Input: part model. Units: mm. Frame: model coordinates. A direction names the side the tool comes from. Round coordinates to 2 decimals unless told otherwise and drop trailing zeros. Write each loop counter-clockwise with the first axis right and the second up, starting at its lowest first coordinate (ties: lowest second). Pieces come first, ordered by that corner, then holes. Notation, with made-up numbers: (-4, 79.5) - (11, 79.5) arc R20 ccw to (11, 105.5) - close; hole circle Ø9 at (-1.75, 56). An arc over 180 degrees is marked (long way). One line per item, written item: value. Start each with the question number.
```python
from build123d import *

# Parameters (mm, degrees)
BOSS_EXTRUDE1_DEPTH     = 25.6
SKETCH2_W               = 4.3
SKETCH2_H               = 15.7
CUT_EXTRUDE1_DEPTH      = 3
CUT_EXTRUDE2_REACH      = 52.281
SKETCH3_R               = 1.3
BOSS_EXTRUDE2_START     = -1.6
BOSS_EXTRUDE2_DEPTH     = 1.6
SKETCH6_W               = 20
SKETCH6_H               = 1.7
BOSS_EXTRUDE3_DEPTH     = 3
CHAMFER2_SIZE           = 3
BOSS_EXTRUDE5_DEPTH     = 17
CHAMFER3_SIZE           = 1.6
CUT_EXTRUDE3_REACH      = 52.926
SKETCH9_W               = 18.51367302
SKETCH9_H               = 5.5
LPATTERN1_COUNT         = 4
LPATTERN1_PITCH         = 7
CUT_EXTRUDE4_REACH      = 53.699
SKETCH10_W              = 21
SKETCH10_H              = 4
LPATTERN2_COUNT         = 4
LPATTERN2_PITCH         = 6
SKETCH11_W              = 4.3
SKETCH11_H              = 15.7
CUT_EXTRUDE5_DEPTH      = 20
CHAMFER4_SIZE           = 4.2
CUT_EXTRUDE6_REACH      = 54.653
SKETCH12_W              = 15.8
SKETCH12_H              = 4
LPATTERN3_COUNT         = 3
LPATTERN3_PITCH         = 6
CUT_EXTRUDE7_REACH      = 55.459
CUT_EXTRUDE7_END_RADIUS = 10.65
SKETCH13_W              = 21
SKETCH13_H              = 3.317301245


# Some blends are built 0.0001 mm under size
with BuildPart() as part:
    # Sketch1 → Boss-Extrude1 (new body)
    with BuildSketch(Plane(origin=(0, 0, 0), x_dir=(0, 0, -1), z_dir=(1, 0, 0))):
        with BuildLine():
            Line((-2, 32), (-2, 30))
            Line((-2, 30), (0, 30))
            Line((0, 30), (0, 34))
            Line((0, 34), (-17.35, 34))
            ThreePointArc((-17.35, 34), (-25.835281374, 30.485281374), (-29.35, 22))
            Line((-29.35, 22), (-29.35, 0))
            Line((-29.35, 0), (-23.7, 0))
            Line((-23.7, 0), (-23.7, 15.7))
            Line((-23.7, 15.7), (-28, 15.7))
            Line((-28, 15.7), (-28, 22))
            ThreePointArc((-28, 22), (-26.080424321, 28.099359898), (-21.01367302, 32))
            Line((-21.01367302, 32), (-2, 32))
        make_face()
    extrude(amount=-BOSS_EXTRUDE1_DEPTH)

    # Sketch2 → Cut-Extrude1 (cut)
    with BuildSketch(Plane(origin=(0, 0, 0), x_dir=(0, 0, -1), z_dir=(1, 0, 0))):
        with Locations((-25.85, 7.85)):
            Rectangle(SKETCH2_W, SKETCH2_H)
    extrude(amount=-CUT_EXTRUDE1_DEPTH, mode=Mode.SUBTRACT)

    # Sketch3 → Cut-Extrude2 (cut, up to next)
    with BuildSketch(Plane(origin=(-3, 0, 0), x_dir=(0, 0, -1), z_dir=(1, 0, 0)), mode=Mode.PRIVATE) as cut_extrude2_sk1:
        with Locations((-25.65, 9.5)):
            Circle(SKETCH3_R)
    cut_extrude2_tool1 = extrude(cut_extrude2_sk1.sketch, amount=-CUT_EXTRUDE2_REACH, mode=Mode.PRIVATE) & part.part
    add(cut_extrude2_tool1.solids().sort_by_distance((-3, 9.5, 25.65))[0], mode=Mode.SUBTRACT)

    # Sketch4 → Boss-Extrude2 (add)
    with BuildSketch(Plane.ZY.offset(25.6).offset(BOSS_EXTRUDE2_START)):
        with BuildLine():
            Line((0, 34), (0, 0))
            Line((0, 0), (29.35, 0))
            Line((29.35, 0), (29.35, 22))
            ThreePointArc((29.35, 22), (25.835281374, 30.485281374), (17.35, 34))
            Line((17.35, 34), (0, 34))
        make_face()
    extrude(amount=BOSS_EXTRUDE2_DEPTH)

    # Sketch6 → Boss-Extrude3 (add)
    with BuildSketch(Plane(origin=(0, 0, 0), x_dir=(-1, 0, 0), z_dir=(0, 0, -1))):
        with Locations((10, 30.85)):
            Rectangle(SKETCH6_W, SKETCH6_H)
    extrude(amount=BOSS_EXTRUDE3_DEPTH)

    # Chamfer2
    chamfer2_edges = [part.edges().sort_by_distance(p)[0] for p in [
        (-20, 30.85, -3),
    ]]
    chamfer(chamfer2_edges, length=CHAMFER2_SIZE - 0.0001)  # a hair under: the kernel refuses the full size

    # Sketch8 → Boss-Extrude5 (add)
    with BuildSketch(Plane.ZY):
        Polygon((-1.408034607, 31.7), (-1.808034607, 33.3), (-3, 33.3), (-3, 31.7), align=None)
    extrude(amount=BOSS_EXTRUDE5_DEPTH)

    # Chamfer3
    chamfer3_edges = [part.edges().sort_by_distance(p)[0] for p in [
        (-17, 33.3, -2.404017304),
    ]]
    chamfer(chamfer3_edges, length=CHAMFER3_SIZE - 0.0001)  # a hair under: the kernel refuses the full size

    # Sketch9 → Cut-Extrude3 (cut, up to next)
    with BuildSketch(Plane(origin=(-24, 0, 0), x_dir=(0, 0, -1), z_dir=(1, 0, 0)), mode=Mode.PRIVATE) as cut_extrude3_sk1:
        with Locations((-13.25683651, 27.25)):
            Rectangle(SKETCH9_W, SKETCH9_H)
    cut_extrude3_tool1 = extrude(cut_extrude3_sk1.sketch, amount=-CUT_EXTRUDE3_REACH, mode=Mode.PRIVATE) & part.part
    cut_extrude3 = cut_extrude3_tool1.solids().sort_by_distance((-24, 27.25, 13.256837))[0]
    add(cut_extrude3, mode=Mode.SUBTRACT)

    # LPattern1: Cut-Extrude3 ×4
    with Locations(*[(0, -i * LPATTERN1_PITCH, 0) for i in range(1, LPATTERN1_COUNT)]):
        add(cut_extrude3, mode=Mode.SUBTRACT)

    # Sketch10 → Cut-Extrude4 (cut, up to next)
    with BuildSketch(Plane(origin=(0, 34, 0), x_dir=(1, 0, 0), z_dir=(0, 1, 0)), mode=Mode.PRIVATE) as cut_extrude4_sk1:
        with Locations((-13.5, -6)):
            Rectangle(SKETCH10_W, SKETCH10_H)
    cut_extrude4_tool1 = extrude(cut_extrude4_sk1.sketch, amount=-CUT_EXTRUDE4_REACH, mode=Mode.PRIVATE) & part.part
    cut_extrude4 = cut_extrude4_tool1.solids().sort_by_distance((-13.5, 34, 6))[0]
    add(cut_extrude4, mode=Mode.SUBTRACT)

    # LPattern2: Cut-Extrude4; each copy of Cut-Extrude4 runs up to whatever stops it at its own place
    lpattern2_before = part.part  # the part as the pattern finds it: every copy runs up to it
    lpattern2_cut_extrude4_long = extrude(cut_extrude4_sk1.sketch, amount=-CUT_EXTRUDE4_REACH, mode=Mode.PRIVATE)
    lpattern2_cut_extrude4_tool1 = lpattern2_cut_extrude4_long.moved(Location(Vector(0, 0, 1) * (1 * LPATTERN2_PITCH))) & lpattern2_before
    add(lpattern2_cut_extrude4_tool1.solids().sort_by_distance((-13.5, 34, 12))[0], mode=Mode.SUBTRACT)
    lpattern2_cut_extrude4_tool2 = lpattern2_cut_extrude4_long.moved(Location(Vector(0, 0, 1) * (2 * LPATTERN2_PITCH))) & lpattern2_before
    add(lpattern2_cut_extrude4_tool2.solids().sort_by_distance((-13.5, 34, 18))[0], mode=Mode.SUBTRACT)
    lpattern2_cut_extrude4_tool3 = lpattern2_cut_extrude4_long.moved(Location(Vector(0, 0, 1) * (3 * LPATTERN2_PITCH))) & lpattern2_before
    add(lpattern2_cut_extrude4_tool3.solids().sort_by_distance((-13.5, 34, 24))[0], mode=Mode.SUBTRACT)

    # Sketch11 → Cut-Extrude5 (cut)
    with BuildSketch(Plane(origin=(-24, 0, 0), x_dir=(0, 0, -1), z_dir=(1, 0, 0))):
        with Locations((-25.85, 7.85)):
            Rectangle(SKETCH11_W, SKETCH11_H)
    extrude(amount=CUT_EXTRUDE5_DEPTH, mode=Mode.SUBTRACT)

    # Chamfer4
    # the kernel refuses this chamfer: 4.2 mm, written as the material it adds along each edge
    with BuildSketch(Plane(origin=(-4, 15.7, 28), x_dir=(-0.9996219169112966, 0, 0.02749587661058612), z_dir=(0, -1, 0))) as chamfer4_piece_1_section:
        Polygon((CHAMFER4_SIZE * 0.999621916911, CHAMFER4_SIZE * 0.0274958766106), (-CHAMFER4_SIZE * 0.0274958766106, CHAMFER4_SIZE * 0.999621916911), (0, 0), align=None)
    chamfer4_piece_1 = extrude(amount=15.7, mode=Mode.PRIVATE)
    chamfer4_piece_1 = chamfer4_piece_1 - Plane(origin=(-5.414149403, 9.5, 25.65), x_dir=(0, 0, -1), z_dir=(1, 0, 0)) * Cylinder(1.3, 49, mode=Mode.PRIVATE)
    add(chamfer4_piece_1)

    # Sketch12 → Cut-Extrude6 (cut, up to next)
    with BuildSketch(Plane(origin=(0, 0, 28), x_dir=(-1, 0, 0), z_dir=(0, 0, -1)), mode=Mode.PRIVATE) as cut_extrude6_sk1:
        with Locations((16.1, 5.5)):
            Rectangle(SKETCH12_W, SKETCH12_H)
    cut_extrude6_tool1 = extrude(cut_extrude6_sk1.sketch, amount=-CUT_EXTRUDE6_REACH, mode=Mode.PRIVATE) & part.part
    cut_extrude6 = cut_extrude6_tool1.solids().sort_by_distance((-16.1, 5.5, 28))[0]
    add(cut_extrude6, mode=Mode.SUBTRACT)

    # LPattern3: Cut-Extrude6 ×3
    with Locations(*[(0, i * LPATTERN3_PITCH, 0) for i in range(1, LPATTERN3_COUNT)]):
        add(cut_extrude6, mode=Mode.SUBTRACT)

    # Cut-Extrude7: up to this cylinder (the profile starts outside it)
    cut_extrude7_end = Plane(origin=(-13.5, 22, 17.35), z_dir=(1, 0, 0)) * Cylinder(CUT_EXTRUDE7_END_RADIUS, 133.218, mode=Mode.PRIVATE)
    # Sketch13 → Cut-Extrude7 (cut, up to the surface)
    with BuildSketch(Plane.XY.offset(29.35), mode=Mode.PRIVATE) as cut_extrude7_sk1:
        with Locations((-13.5, 26.158650623)):
            Rectangle(SKETCH13_W, SKETCH13_H)
    cut_extrude7_tool1 = extrude(cut_extrude7_sk1.sketch, amount=-CUT_EXTRUDE7_REACH, mode=Mode.PRIVATE) - cut_extrude7_end
    add(cut_extrude7_tool1.solids().sort_by_distance((-13.5, 26.158651, 29.35))[0], mode=Mode.SUBTRACT)


solid = part.part
```
Q1. Contact query for flat-ended pins moving along their axis: pin 1 Ø8 at (y, z) = (7, 19) entering from +X; pin 2 Ø1.2 at (x, y) = (-12.5, 32.5) entering from +Z; pin 3 Ø15 at (x, z) = (-10, 12) entering from -Y; pin 4 Ø1 at (y, z) = (12.5, 13.5) entering from +X. Output: stop coordinate, or through.
Q2. Access query for faces 1 (the flat face through (-14, 33, 20)), 2 (the flat face through (-25, 24.5, 13)), 3 (the flat face through (-11.8, 32, 9.5)). Directions: +Z, -Z, +X, -X, +Y, -Y. A direction counts if a zero-diameter tool reaches every point of the face in a straight line with its end or side. Return the directions, or none.
Q3. Cut plane D-D, the plane x = -3.5. Count the separate pieces of the cut face and the enclosed holes in it, and give its area (3 significant figures).
Q4. Cut plane A-A, the plane z = 14.5. Output: boundary loops of the cut face in (x, y).
Q5. Cut plane B-B, the plane y = 7. Output: boundary loops of the cut face in (x, z).
Q6. Material intervals for probe 1 along Y at (x, z) = (-5.75, 25.65); probe 2 along Z at (x, y) = (-4.4, 9.5); probe 3 along X at (y, z) = (1, 25), sorted ascending. Write a range as from..to.
Q7. Pull-direction query (Y, two-part tool) for faces 4 (the flat face through (-3, 33, 18)), 5 (the flat face through (-8.381, 32.489, -1.605)), 6 (the flat face through (-25, 10.5, 13)); classes: pulls with the +Y half, pulls with the -Y half, needs draft (parallel to the pull), parting line crosses it, or undercut.
Q8. Cut plane C-C, the plane y = 21. Output: boundary loops of the cut face in (x, z), and give its area (3 significant figures).
A:
1. pin 1: stops at x = -24
1. pin 2: stops at z = 22
1. pin 3: stops at y = 32
1. pin 4: passes through
2. face 1: +Y, -Y
2. face 2: +X, -X
2. face 3: +X, -Y
3. separate pieces: 6
3. enclosed holes: 1
3. area: 128 mm²
4. outline: (-25.6, 0) - (-24, 0) - (-24, 3.5) - (-25.6, 3.5) - close; (-25.6, 9) - (-24, 9) - (-24, 10.5) - (-25.6, 10.5) - close; (-25.6, 16) - (-24, 16) - (-24, 17.5) - (-25.6, 17.5) - close; (-25.6, 23) - (-24, 23) - (-24, 24.5) - (-25.6, 24.5) - close; (-25.6, 30) - (-24, 30) - (-24, 32) - (0, 32) - (0, 34) - (-25.6, 34) - close
5. outline: (-25.6, 0) - (-24, 0) - (-24, 4) - (-25.6, 4) - close; (-25.6, 22.51) - (-24, 22.51) - (-24, 29.35) - (-25.6, 29.35) - close; (-8.2, 28) - (-4, 23.8) - (-4, 23.7) - (-3, 23.7) - (-3, 28) - (0, 28) - (0, 29.35) - (-8.2, 29.35) - close
6. probe 1: y = 0..8.2, 10.8..15.7
6. probe 2: z = 24.2..24.35, 26.95..29.35
6. probe 3: x = -25.6..-24, -5.2..-3
7. face 4: needs draft
7. face 5: pulls with the +Y half
7. face 6: undercut
8. outline: (-25.6, 0) - (-24, 0) - (-24, 4) - (-25.6, 4) - close; (-25.6, 22.51) - (-24, 22.51) - (-24, 28) - (0, 28) - (0, 29.35) - (-25.6, 29.35) - close
8. area: 49.7 mm²
